Autodesk Inventor part; units mm, degrees
ref_plane "YZ Plane" through (0, 0, 0) normal (1, 0, 0) x (0, 1, 0)
ref_plane "XZ Plane" through (0, 0, 0) normal (0, 1, 0) x (-1, 0, 0)
ref_plane "XY Plane" through (0, 0, 0) normal (0, 0, 1) x (1, 0, 0)
sketch "Sketch1" plane through (0, 0, 0) normal (0, 0, 1) x (1, 0, 0)
  circle A0 centre (0, 0) radius 18.8087
  circle A1 centre (0, 0) radius 20.6375
  dimension "d0" = 37.6174
  dimension "d1" = 41.275
extrude "Extrusion1" add sketch "Sketch1" along normal blind 300
ref_plane "Work Plane1" through (-18.8087, 0, 0) normal (0, -1, 0) x (1, 0, 0)
sketch "Sketch3" plane through (-18.8087, 0, 0) normal (0, -1, 0) x (1, 0, 0)
  line L0 (18.8087, 0) -> (18.8087, 150)
  line L1 (18.8087, 0) -> (18.8087, 300)
  line L2 (18.8087, 150) -> (18.8087, 90)
  line L3 (18.8087, 90) -> (18.8087, 210)
  line L4 (18.8087, 90) -> (18.8087, 85)
  line L5 (18.8087, 210) -> (18.8087, 215)
  circle A0 centre (18.8087, 215) radius 2.5
  circle A1 centre (18.8087, 85) radius 2.5
  dimension "d6" = 150
  dimension "d7" = 60
  dimension "d8" = 120
  dimension "d9" = 5
  dimension "d10" = 5
  dimension "d11" = 5
  dimension "d12" = 5
extrude "Extrusion3" cut sketch "Sketch3" along normal mid plane 300
properties part number "4000_Cu_Bias_Shielding_(McMaster_50475K18)_MPSv2_v1" material "Copper"
CAD build for the part. Positions are in the model's coordinates, mm. Round coordinates to 2 decimals unless told otherwise and drop trailing zeros. Order: outer loops, then holes, each group sorted by start corner. A loop starts at its lowest first (then second) coordinate and runs counter-clockwise, first axis right, second up.
Item 1: Saw through at A-A on y = 0. Write the cut outline in (x, z), then the cut area to 3 significant figures.
Item 2: Pin check, flat tips, straight feed: pin 1 (5 mm diameter, centred on y = 6.5, z = 165.5, fed in from -X); pin 2 (4 mm diameter, centred on x = -5.5, z = 99, fed in from -Y); pin 3 (8 mm diameter, centred on x = 0, z = 215, fed in from +Y); pin 4 (5 mm diameter, centred on x = -7, z = 256, fed in from +Y). Stop position of each tip, or through.
Item 3: Mould opens along Y. For faces 1 (the face through (-2.5, 19.6, 215.1)), 2 (the face through (-4.474, 20.147, 147.9)), 3 (the face through (-4.08, 18.36, 147.9)) say: pulls with the +Y half, pulls with the -Y half, needs draft (parallel to the pull), parting line crosses it, or undercut.
Item 4: Probe line 1 along Y through (x, z) = (0, 104); line 2 along Z through (x, y) = (0, 19.65); line 3 along X through (y, z) = (2, 247). List the from-to ranges inside material, lowest first.
Item 5: Saw through at B-B on x = 0. Write the cut outline in (y, z), then the cut area to 3 significant figures.
Reported:
1. outline: (-20.64, 0) - (-18.81, 0) - (-18.81, 300) - (-20.64, 300) - close; (18.81, 0) - (20.64, 0) - (20.64, 300) - (18.81, 300) - close
1. area: 1,100 mm2
2. pin 1: stops at x = -20.25
2. pin 2: stops at y = -20.34
2. pin 3: stops at y = 20.64
2. pin 4: stops at y = 20.14
3. face 1: needs draft
3. face 2: parting line crosses it
3. face 3: undercut
4. line 1: y = -20.64 to -18.81, 18.81 to 20.64
4. line 2: z = 0 to 82.5, 87.5 to 212.5, 217.5 to 300
4. line 3: x = -20.54 to -18.7, 18.7 to 20.54
5. outline: (-20.64, 0) - (-18.81, 0) - (-18.81, 82.5) - (-20.64, 82.5) - close; (-20.64, 87.5) - (-18.81, 87.5) - (-18.81, 212.5) - (-20.64, 212.5) - close; (-20.64, 217.5) - (-18.81, 217.5) - (-18.81, 300) - (-20.64, 300) - close; (18.81, 0) - (20.64, 0) - (20.64, 82.5) - (18.81, 82.5) - close; (18.81, 87.5) - (20.64, 87.5) - (20.64, 212.5) - (18.81, 212.5) - close; (18.81, 217.5) - (20.64, 217.5) - (20.64, 300) - (18.81, 300) - close
5. area: 1,060 mm2
